Autodesk Inventor part; units mm, degrees
ref_plane "YZ Plane" through (0, 0, 0) normal (1, 0, 0) x (0, 1, 0)
ref_plane "XZ Plane" through (0, 0, 0) normal (0, 1, 0) x (-1, 0, 0)
ref_plane "XY Plane" through (0, 0, 0) normal (0, 0, 1) x (1, 0, 0)
sketch "Sketch1" plane through (0, 0, 0) normal (0, 1, 0) x (-1, 0, 0)
  line L0 (0, 0) -> (25.4, 0)
  line L1 (25.4, 0) -> (25.4, -76.2)
  line L2 (25.4, -76.2) -> (0, -76.2)
  line L3 (0, -76.2) -> (0, 0)
  line L4 (0, 0) -> (76.2, 0)
  line L5 (76.2, 0) -> (76.2, -25.4)
  line L6 (76.2, -25.4) -> (0, -25.4)
  line L7 (0, -25.4) -> (0, 0)
  line L8 (76.2, -12.7) -> (0, -12.7)
  line L9 (12.7, -76.2) -> (12.7, 0)
  line L10 (12.7, -12.7) -> (38.1, -12.7)
  line L11 (38.1, -12.7) -> (63.5, -12.7)
  line L12 (12.7, -12.7) -> (12.7, -38.1)
  line L13 (12.7, -38.1) -> (12.7, -63.5)
  circle A0 centre (12.7, -12.7) radius 3.81
  circle A1 centre (38.1, -12.7) radius 3.81
  circle A2 centre (63.5, -12.7) radius 3.81
  circle A3 centre (12.7, -38.1) radius 3.81
  circle A4 centre (12.7, -63.5) radius 3.81
  line L14 (76.2, -25.4) -> (25.4, -76.2)
  point P0 (25.4, -25.4)
  dimension "d0" = 25.4
  dimension "d1" = 76.2
  dimension "d2" = 76.2
  dimension "d3" = 25.4
  dimension "d4" = 25.4
  dimension "d5" = 25.4
  dimension "d6" = 25.4
  dimension "d7" = 25.4
  dimension "d8" = 7.62
  dimension "d9" = 7.62
  dimension "d10" = 7.62
  dimension "d11" = 7.62
  dimension "d12" = 7.62
extrude "Extrusion1" add sketch "Sketch1" along normal blind 5.08 contours L0 L9 A0 L8 L3 | L0 L1 L8 A0 L9 | L8 A0 L9 L6 L3 | L4 L5 L8 A2 A1 L1 | L6 L9 A3 A4 L2 L3 | L8 A1 A2 L5 L6 L1 | L1 L6 L9 A0 L8 | L6 L1 L2 L9 A4 A3 | L6 L14 L1
equation "\"d9\" = d8"
equation "\"d10\" = d8"
equation "\"d11\" = d8"
equation "\"d12\" = d8"
properties part number "corner_bracket" material "Aluminum 6061"
Source: CAD feature listing. Evaluate the final solid. Frame: model axes, mm. Round coordinates to 2 decimals unless told otherwise and drop trailing zeros. Order: outer loops, then holes, each group sorted by start corner. A loop starts at its lowest first (then second) coordinate and runs counter-clockwise, first axis right, second up. Notation, with made-up numbers: (2, 81) - (23, 81) arc R14 cw to (23, 98) - close; hole circle Ø5 at (-3, 80.5). An arc over 180 degrees is marked (long way). Use a Markdown table: item, result. Add a question column.
1. Mould query, pull axis X, two halves, no side actions, for faces 1 (the flat face through (0, 3, -39)), 2 (the flat face through (-76.2, 3, -13)), 3 (the cylindrical face through (-34.294, 2.504, -12.868)). Classes: +X half, -X half, draft (parallel to the pull), parting line (faces both ways), or undercut.
2. Section query A-A (x = -38.1). Return the cut outline in (y, z).
3. First-contact query: pin 1 (3 mm diameter, centred on y = 2, z = -29.5, fed in from -X). Flat tip, straight axial feed; report the tip coordinate or a pass-through.
4. Section query C-C (x = -12.7). Return the cut outline in (y, z).
5. Line query: probe 1 along Z at (x, y) = (-12.7, 3.1); probe 2 along X at (y, z) = (1.5, -10). Output: solid intervals per line, ascending.
6. Section query B-B (z = -12.7). Return the cut outline in (x, y), then the cut area to 3 significant figures.
7. Section query D-D (y = 1.5). Return the cut outline in (x, z), then the cut area to 3 significant figures.
Derived:
| question | item | result |
|---|---|---|
| 1 | face 1 | +X half |
| 1 | face 2 | -X half |
| 1 | face 3 | undercut |
| 2 | outline | (0, -63.5) - (5.08, -63.5) - (5.08, -16.51) - (0, -16.51) - close; (0, -8.89) - (5.08, -8.89) - (5.08, 0) - (0, 0) - close |
| 3 | pin 1 | x = -73.6 |
| 4 | outline | (0, -76.2) - (5.08, -76.2) - (5.08, -67.31) - (0, -67.31) - close; (0, -59.69) - (5.08, -59.69) - (5.08, -41.91) - (0, -41.91) - close; (0, -34.29) - (5.08, -34.29) - (5.08, -16.51) - (0, -16.51) - close; (0, -8.89) - (5.08, -8.89) - (5.08, 0) - (0, 0) - close |
| 5 | probe 1 | -76.2 to -67.31, -59.69 to -41.91, -34.29 to -16.51, -8.89 to 0 |
| 5 | probe 2 | -76.2 to -66.19, -60.81 to -40.79, -35.41 to -15.39, -10.01 to 0 |
| 6 | outline | (-76.2, 0) - (-67.31, 0) - (-67.31, 5.08) - (-76.2, 5.08) - close; (-59.69, 0) - (-41.91, 0) - (-41.91, 5.08) - (-59.69, 5.08) - close; (-34.29, 0) - (-16.51, 0) - (-16.51, 5.08) - (-34.29, 5.08) - close; (-8.89, 0) - (0, 0) - (0, 5.08) - (-8.89, 5.08) - close |
| 6 | area | 271 mm2 |
| 7 | outline | (-76.2, -25.4) - (-25.4, -76.2) - (0, -76.2) - (0, 0) - (-76.2, 0) - close; hole circle Ø7.62 at (-63.5, -12.7); hole circle Ø7.62 at (-38.1, -12.7); hole circle Ø7.62 at (-12.7, -63.5); hole circle Ø7.62 at (-12.7, -38.1); hole circle Ø7.62 at (-12.7, -12.7) |
| 7 | area | 4,290 mm2 |
